Input: part model. Units: mm. Frame: model coordinates. A direction names the side the tool comes from. Give positions to 0.01 mm unless a question says otherwise; leave off trailing zeros. Order: outer loops, then holes, each group sorted by start corner. A loop starts at its lowest first (then second) coordinate and runs counter-clockwise, first axis right, second up. Notation, with made-up numbers: M 32.5,-9.75 L 61.5,-9.75 A17 cw 61.5,-0.75 Z; hole C -3.5,21.5 d7. An arc over 180 degrees is marked long. Use a Markdown table: item, result.
from build123d import *

# Parameters (mm, degrees)
F2_R     = 6
F3_DEPTH = 25
F4_R     = 33.7409795254
F4_R_2   = 6
F5_DEPTH = 25


with BuildPart() as f1:
    # F0 (on Front) → F1 (revolve)
    with BuildSketch(Plane.XZ):
        with BuildLine():
            Line((12.1142669689, 0), (12.1142669689, 182.7975656304))
            ThreePointArc((12.1142669689, 182.7975656304), (0, 210.5), (-12.1142669689, 182.7975656304))
            Line((-12.1142669689, 182.7975656304), (-12.1142669689, 0))
            Line((-12.1142669689, 0), (12.1142669689, 0))
        make_face()
    revolve(axis=Axis((0, 0, 0), (1, 0, 0)))

    # F2 (on face) → F3 (cut)
    with BuildSketch(Plane.YZ.offset(12.1142669689)):
        Circle(F2_R)
    extrude(amount=-F3_DEPTH, mode=Mode.SUBTRACT)

    # F4 (on Right) → F5 (join, symmetric)
    with BuildSketch(Plane.YZ):
        Circle(F4_R)
        Circle(F4_R_2, mode=Mode.SUBTRACT)
    extrude(amount=F5_DEPTH, both=True)


solid = f1.part
1) Cut plane A-A on y = 0. Return loops of the section in (x, z).
Response values:
| item | result |
|---|---|
| outline | M -25,-33.74 L -12.11,-33.74 L -12.11,-182.8 A16.5 ccw long 12.11,-182.8 L 12.11,-33.74 L 25,-33.74 L 25,-6 L -25,-6 Z; M -25,6 L 25,6 L 25,33.74 L 12.11,33.74 L 12.11,182.8 A16.5 ccw long -12.11,182.8 L -12.11,33.74 L -25,33.74 Z |
2) Material intervals for line 1 (Z direction, x = 0, y = 0); line 2 (Z direction, x = -14, y = 0); line 3 (Z direction, x = 8.5, y = 0), sorted ascending. Write a range as from..to.
Response values:
| item | result |
|---|---|
| line 1 | z = -210.5..-6, 6..210.5 |
| line 2 | z = -202.73..-185.27, -33.74..-6, 6..33.74, 185.27..202.73 |
| line 3 | z = -208.14..-6, 6..208.14 |
3) Reachability of faces 1 (the face through (12.114, 38, 3)), 2 (the face through (-12.114, 38, -3)), 3 (the face through (25, 7, 0)) from +Z, -Z, +X, -X, +Y, -Y: full face, straight path, thin tool, end or side. Return the list, or none.
Response values:
| item | result |
|---|---|
| face 1 | +X |
| face 2 | -X |
| face 3 | +Z, -Z, +X, +Y, -Y |
4) Cut plane C-C on x = -1. Return loops of the section in (y, z), and give its area (3 significant figures).
Response values:
| item | result |
|---|---|
| outline | C 0,0 d420.94; hole C 0,0 d12 |
| area | 139,000 mm² |
5) First-contact query: pin 1 Ø2 at (y, z) = (121.5, 64) entering from +X; pin 2 Ø1 at (x, y) = (13, 143.5) entering from +Z; pin 3 Ø4 at (y, z) = (9.5, -87) entering from -X; pin 4 Ø9.5 at (y, z) = (0, 0) entering from +X. Flat tips, straight axial feed; report the tip coordinate or a pass-through.
Response values:
| item | result |
|---|---|
| pin 1 | stops at x = 12.11 |
| pin 2 | stops at z = 146.21 |
| pin 3 | stops at x = -12.11 |
| pin 4 | passes through |
